Design review of the part built by this model. Coordinates are the model's own, in mm. A direction names the side the tool comes from. Coordinates: 2 decimals unless noted, no trailing zeros. Write each loop counter-clockwise with the first axis right and the second up, starting at its lowest first coordinate (ties: lowest second). Pieces come first, ordered by that corner, then holes. Notation, with made-up numbers: M -33,-11 L -25,-11 A14 cw -25,0 Z; hole C 58.25,24.25 d8. An arc over 180 degrees is marked long. Write item = value, one per line.
Autodesk Inventor part; units mm, degrees
ref_plane "b6000_1_XY" through (7, 0, 0) normal (1, 0, 0) x (0, 0, -1)
ref_plane "b6000_1_YZ" through (7, 0, 0) normal (0, 0, -1) x (0, 1, 0)
ref_plane "b6000_1_ZX" through (7, 0, 0) normal (0, 1, 0) x (1, 0, 0)
sketch "_____1" plane through (0, 0, 0) normal (0, 0, 1) x (1, 0, 0)
  line L0 (11, 0) -> (-11, 0)
  line L1 (-11, 0) -> (-11, 17.5)
  line L2 (-11, 17.5) -> (11, 17.5)
  line L3 (11, 17.5) -> (11, 0)
  line L4 (11, 0) -> (-11, 0)
revolve "Revolution1" add sketch "_____1" angle 360 about axis through (11, 0, 0) along (1, 0, 0)
sketch "_____3" plane through (0, 0, 0) normal (0, 0, 1) x (1, 0, 0)
  line L0 (11, 0) -> (-11, 0)
  line L1 (-11, 0) -> (-11, 13)
  line L2 (-11, 13) -> (-3, 13)
  line L3 (-3, 13) -> (-3, 11.5)
  line L4 (-3, 11.5) -> (3, 11.5)
  line L5 (3, 11.5) -> (3, 13)
  line L6 (3, 13) -> (11, 13)
  line L7 (11, 13) -> (11, 0)
  line L8 (11, 0) -> (-11, 0)
revolve "Revolution2" cut sketch "_____3" angle 360 about axis through (11, 0, 0) along (1, 0, 0)
ref_plane "b6000_1_XY" through (7, 0, 0) normal (1, 0, 0) x (0, 0, -1)
ref_plane "b6000_1_YZ" through (7, 0, 0) normal (0, 0, -1) x (0, 1, 0)
ref_plane "b6000_1_ZX" through (7, 0, 0) normal (0, 1, 0) x (1, 0, 0)
ref_plane "b6000_2_XY" through (-7, 0, 0) normal (1, 0, 0) x (0, 0, -1)
ref_plane "b6000_2_YZ" through (-7, 0, 0) normal (0, 0, -1) x (0, 1, 0)
ref_plane "b6000_2_ZX" through (-7, 0, 0) normal (0, 1, 0) x (1, 0, 0)
ref_plane "to_dummy_XY" through (0, 0, 0) normal (1, 0, 0) x (0, 0, -1)
ref_plane "to_dummy_YZ" through (0, 0, 0) normal (0, 0, -1) x (0, 1, 0)
ref_plane "to_dummy_ZX" through (0, 0, 0) normal (0, 1, 0) x (1, 0, 0)
properties part number "C-AFBD22-35W_bw"
Q1. Machinability: for faces 5 (the flat face through (3, 5, -11)), 6 (the flat face through (-11, -3, 13)), 7 (the cylindrical face through (-6.944, -10.316, -7.91)), which of the approach directions +Z, -Z, +X, -X, +Y, -Y give a long, thin tool a straight path to every point of the face, cutting with its end or side? Answer none if there is none.
Check result:
face_5 = +X
face_6 = +Z, -Z, -X, +Y, -Y
face_7 = -X
Q2. Consider section D-D, the plane z = 14. State the section outline as (x, y) points, and give its area (3 significant figures).
Check result:
outline = M -11,-10.5 L 11,-10.5 L 11,10.5 L -11,10.5 Z
area = 462 mm²
Q3. Wall thickness on line 1 (Z direction, x = 5, y = 0); line 2 (Z direction, x = 0.3, y = 0); line 3 (Y direction, x = -3.25, z = -12): over which ranges is each line inside the solid? List them lowest first.
Check result:
line_1 = -17.5 to -13, 13 to 17.5
line_2 = -17.5 to -11.5, 11.5 to 17.5
line_3 = -12.74 to -5, 5 to 12.74
Q4. Consider section C-C, the plane x = 0. State the section outline as (y, z) points.
Check result:
outline = C 0,0 d35; hole C 0,0 d23
Q5. For P1, Ø1.5, axis at x = -6.5, y = -7, coming from the +Z side; P2, Ø10, axis at y = -6, z = -4, coming from the -X side; P3, Ø6, axis at x = -7, y = 4.5, coming from the -Z side; P4, Ø13, axis at y = -1, z = 3, coming from the -X side, all flat-tipped, find the tip position at first contact; note any pin that passes through.
Check result:
P1 = 16.35
P2 = -3
P3 = -17.44
P4 = through
Q6. The part is to be moulded in two halves that separate along Z. For faces 1 (the flat face through (11, -3, 13)), 2 (the cylindrical face through (0.154, -13.887, -10.648)), 3 (the cylindrical face through (7.056, -10.316, -7.91)), 4 (the cylindrical face through (0, -1.5, 11.4)), say which applies: +Z half, -Z half, draft (parallel to the pull), parting line (faces both ways), or undercut.
Check result:
face_1 = draft
face_2 = parting line
face_3 = undercut
face_4 = undercut
Q7. Consider section A-A, the plane y = 0. State the section outline as (x, z) points.
Check result:
outline = M -11,-17.5 L 11,-17.5 L 11,-13 L 3,-13 L 3,-11.5 L -3,-11.5 L -3,-13 L -11,-13 Z; M -11,13 L -3,13 L -3,11.5 L 3,11.5 L 3,13 L 11,13 L 11,17.5 L -11,17.5 Z
